The drawing under review shows one solid part. Ordinate dimensions are in mm from its lowest x, y, z. Round coordinates to 2 decimals unless told otherwise and drop trailing zeros. Order: outer loops, then holes, each group sorted by start corner. A loop starts at its lowest first (then second) coordinate and runs counter-clockwise, first axis right, second up. Notation, with made-up numbers: M 20,66.5 L 35,66.5 A30 cw 35,99.5 Z; hole C 41.5,70 d5. An arc over 180 degrees is marked long. Answer as a JSON object with one key per item and string values.
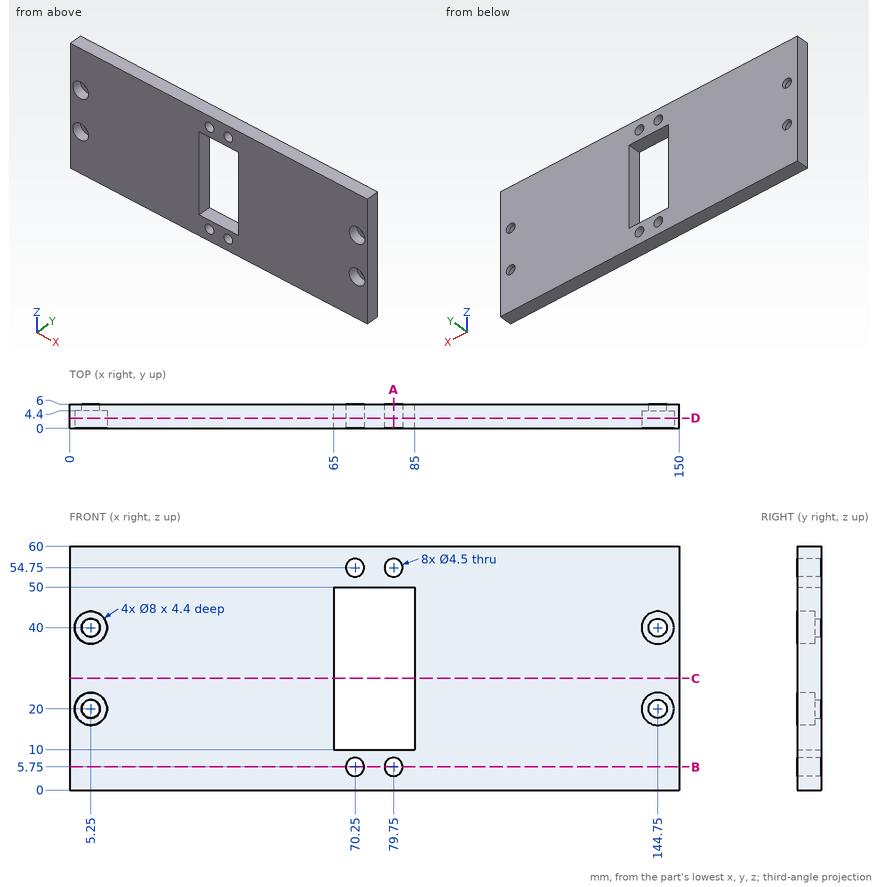
1) Add section A-A on x = 79.75. State the section outline as (y, z) points, and give its area (3 significant figures).
Geometry check:
{"outline": "M 0,0 L 6,0 L 6,3.5 L 0,3.5 Z; M 0,8 L 6,8 L 6,10 L 0,10 Z; M 0,50 L 6,50 L 6,52.5 L 0,52.5 Z; M 0,57 L 6,57 L 6,60 L 0,60 Z", "area": "66.0 mm²"}
2) Add section D-D on y = 2.5. State how many separate pieces and enclosed holes the cut face has, and give its area (3 significant figures).
Geometry check:
{"separate pieces": "1", "enclosed holes": "9", "area": "7,940 mm²"}
3) Insertion check: P1, Ø3.5, axis at x = 5.25, z = 40, coming from the +Y side; P2, Ø2.5, axis at x = 145, z = 21, coming from the -Y side. Each pin has a flat end and moves straight along its axis. Give the tip position at first contact, or say it passes through.
Geometry check:
{"P1": "passes through", "P2": "stops at y = 4.4"}
4) Add section B-B on z = 5.75. State the section outline as (x, y) points.
Geometry check:
{"outline": "M 0,0 L 68,0 L 68,6 L 0,6 Z; M 72.5,0 L 77.5,0 L 77.5,6 L 72.5,6 Z; M 82,0 L 150,0 L 150,6 L 82,6 Z"}
5) For L1, parallel to Z at x = 5.25, y = 1.6; L2, parallel to X at y = 1.4, z = 54.75; L3, parallel to Z at x = 70.25, y = 1.4, list the stretches that pass through material, from the lowest coordinate up.
Geometry check:
{"L1": "z = 0 to 16, 24 to 36, 44 to 60", "L2": "x = 0 to 68, 72.5 to 77.5, 82 to 150", "L3": "z = 0 to 3.5, 8 to 10, 50 to 52.5, 57 to 60"}
6) Add section C-C on z = 27.5. State the section outline as (x, y) points.
Geometry check:
{"outline": "M 0,0 L 65,0 L 65,6 L 0,6 Z; M 85,0 L 150,0 L 150,6 L 85,6 Z"}
